```python
from build123d import *

# Parameters (mm, degrees)
F0_W       = 25.4
F0_H       = 25.4
F1_DEPTH   = 381
F2_SIZE2   = 10.521014
F2_SIZE    = 25.39999
F2_2_SIZE2 = 10.521014
F2_2_SIZE  = 25.39999


# Not quite as in the source:
# - a fillet or chamfer is up to 0.001 mm smaller than in the source, because OpenCascade refuses the exact size


with BuildPart() as f1:
    # F0 (on Front) → F1 (new body, symmetric)
    with BuildSketch(Plane.XZ):
        Rectangle(F0_W, F0_H)
    extrude(amount=F1_DEPTH, both=True)

    # F2 (size 25.4 and 10.5210244843 in the source; OpenCascade refuses exactly that, so slightly less here)
    f2_edges = [f1.edges().sort_by_distance(p)[0] for p in [
        (12.7, -381, 0),
    ]]
    f2_side = f1.faces().sort_by_distance((0, -381, 0))[0]
    chamfer(f2_edges, length=F2_SIZE, length2=F2_SIZE2, reference=f2_side)

    # F2#2 (size 25.4 and 10.5210244843 in the source; OpenCascade refuses exactly that, so slightly less here)
    f2_2_edges = [f1.edges().sort_by_distance(p)[0] for p in [
        (12.7, 381, 0),
    ]]
    f2_2_side = f1.faces().sort_by_distance((0, 381, 0))[0]
    chamfer(f2_2_edges, length=F2_2_SIZE, length2=F2_2_SIZE2, reference=f2_2_side)


solid = f1.part
```
The model under review builds one solid part; all positions refer to its coordinate system, in mm. Round coordinates to 2 decimals unless told otherwise and drop trailing zeros. Loops run counter-clockwise (first coordinate to the right, second up) from the corner with the lowest first, then second, coordinate; pieces in that order, holes last. Notation, with made-up numbers: (-19.5, 65) - (1.5, 65) arc R20 ccw to (1.5, 98) - close; hole circle Ø6 at (65, 25.25). An arc over 180 degrees is marked (long way). Use a Markdown table: item, result. Add a question column.
Q1. Add section A-A (x = 6.5). State the section outline as (y, z) points.
Q2. Insertion check: pin 1 Ø12 at (x, z) = (8, -7) entering from +Y; pin 2 Ø4 at (x, z) = (5.5, -1.5) entering from +Y; pin 3 Ø8 at (x, z) = (-6, 2.5) entering from +Y. Each pin has a flat end and moves straight along its axis. Give the tip position at first contact, or say it passes through.
Q3. For probe 1 along Y at (x, z) = (5, 1); probe 2 along Y at (x, z) = (-4, -2.25), list the stretches that pass through material, from the lowest coordinate up.
Worked answers:
| question | item | result |
|---|---|---|
| 1 | outline | (-373.05, -12.7) - (373.05, -12.7) - (373.05, 12.7) - (-373.05, 12.7) - close |
| 2 | pin 1 | y = 374.91 |
| 2 | pin 2 | y = 374.29 |
| 2 | pin 3 | y = 379.88 |
| 3 | probe 1 | -373.67 to 373.67 |
| 3 | probe 2 | -377.4 to 377.4 |
